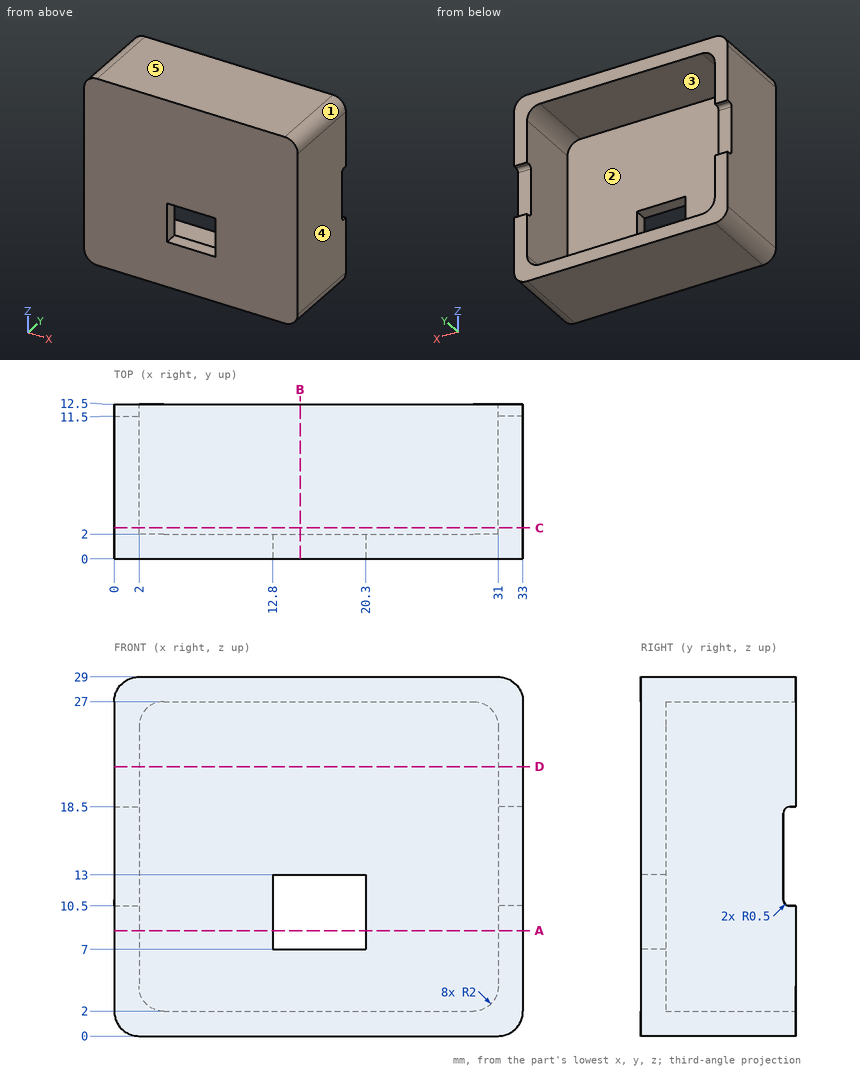
For this review, use the dimensioned drawing (mm, ordinates from the lowest corner) and the shaded views. A direction names the side the tool comes from. Round coordinates to 2 decimals unless told otherwise and drop trailing zeros. Order: outer loops, then holes, each group sorted by start corner. A loop starts at its lowest first (then second) coordinate and runs counter-clockwise, first axis right, second up.
1) Clearance check with flat-ended pins moving along their axes: pin 1 Ø7.5 at (x, z) = (17.5, 11) entering from +Y; pin 2 Ø0.6 at (x, z) = (0.5, 14) entering from +Y. State where each tip first meets the part, or that it passes through.
The answers:
pin 1: stops at y = 2
pin 2: stops at y = 11.5
2) For L1, parallel to X at y = 10, z = 23; L2, parallel to Z at x = 12, y = 9.75; L3, parallel to Y at x = 26.5, z = 21.5, list the stretches that pass through material, from the lowest coordinate up.
The answers:
L1: x = 0 to 2, 31 to 33
L2: z = 0 to 2, 27 to 29
L3: y = 0 to 2
3) Consider section D-D (z = 21.75). State the section outline as (x, y) points.
The answers:
outline: (0, 0) - (33, 0) - (33, 12.5) - (31, 12.5) - (31, 2) - (2, 2) - (2, 12.5) - (0, 12.5) - close
4) Draft analysis for pull direction Z (two halves, no side actions). For the marked faces 3, 4 and 5, state which applies: released by +Z, released by -Z, zero draft, split by the parting line, or undercut.
The answers:
face 3: undercut
face 4: zero draft
face 5: released by +Z
5) Machinability: for the marked faces 1 and 2, which of the approach directions +Z, -Z, +X, -X, +Y, -Y give a long, thin tool a straight path to every point of the face, cutting with its end or side? Answer none if there is none.
The answers:
face 1: +Z, +X, +Y, -Y
face 2: +Y
6) Consider section B-B (x = 15). State the section outline as (y, z) points, plus the area to 3 significant figures.
The answers:
outline: (0, 0) - (12.5, 0) - (12.5, 2) - (2, 2) - (2, 7) - (0, 7) - close; (0, 13) - (2, 13) - (2, 27) - (12.5, 27) - (12.5, 29) - (0, 29) - close
area: 88.0 mm2
7) Consider section A-A (z = 8.5). State the section outline as (x, y) points, plus the area to 3 significant figures.
The answers:
outline: (0, 0) - (12.8, 0) - (12.8, 2) - (2, 2) - (2, 12.5) - (0, 12.5) - close; (20.3, 0) - (33, 0) - (33, 12.5) - (31, 12.5) - (31, 2) - (20.3, 2) - close
area: 93.0 mm2
8) Consider section C-C (y = 2.5). State the section outline as (x, z) points, plus the area to 3 significant figures.
The answers:
outline: (0, 2) arc R2 ccw to (2, 0) - (31, 0) arc R2 ccw to (33, 2) - (33, 27) arc R2 ccw to (31, 29) - (2, 29) arc R2 ccw to (0, 27) - close; hole (2, 4) arc R2 ccw to (4, 2) - (29, 2) arc R2 ccw to (31, 4) - (31, 25) arc R2 ccw to (29, 27) - (4, 27) arc R2 ccw to (2, 25) - close
area: 232 mm2
